The model under review builds one solid part; all positions refer to its coordinate system, in mm. A direction names the side the tool comes from. Coordinates: 2 decimals unless noted, no trailing zeros. Write each loop counter-clockwise with the first axis right and the second up, starting at its lowest first coordinate (ties: lowest second). Pieces come first, ordered by that corner, then holes.
```python
from build123d import *

# Parameters (mm, degrees)
F0_W        = 50
F0_H        = 40
F1_DEPTH    = 8
F2_T        = -1
F3_W        = 15.0767099112
F3_H        = 12.3402951285
F4_DEPTH    = 10
F5_T        = 0.5
F5_T3_DEPTH = 8
F5_T5_DEPTH = 49
F5_T7_DEPTH = 39


# Not quite as in the source:
# - a shell that OpenCascade refuses in one call is made with other operations: the cavity is built on its own and cut out


with BuildPart() as f1:
    # F0 (on Front) → F1 (new body)
    with BuildSketch(Plane.XZ):
        with Locations((-5.8206513731, 0.1503955573)):
            Rectangle(F0_W, F0_H)
    extrude(amount=F1_DEPTH)

    # F2
    f2_openings = [f1.faces().sort_by_distance(p)[0] for p in [
        (-5.820651, 0, 0.150396),
    ]]
    offset(amount=F2_T, openings=f2_openings)

    # F3 (on face) → F4 (join)
    with BuildSketch(Plane(origin=(0, -7, 0), x_dir=(-1, 0, 0), z_dir=(0, 1, 0))):
        with Locations((7.5383549556, -0.1530931331)):
            Rectangle(F3_W, F3_H)
    extrude(amount=F4_DEPTH)

    # F5: shell of thickness 0.5, made by hand


with BuildPart() as f5_core1:
    # F5_t2: copy of F1
    add(f1.part)

    # the walls: a layer under each face that stays
    f5_faces = [f5_core1.faces().sort_by_distance(p)[0] for p in [
        (-5.8206513731, -4, 20.1503955573),
        (19.1793486269, -4, 0.1503955573),
        (-30.8206513731, -4, 0.1503955573),
        (11.3668486269, 0, -19.3557772822),
        (-5.8206513731, -8, 0.1503955573),
        (-5.8206513731, -4, -19.8496044427),
        (-5.8206513731, -3.5, 19.1503955573),
        (18.1793486269, -3.5, 0.1503955573),
        (-5.8206513731, -3.5, -18.8496044427),
        (-29.8206513731, -3.5, 0.1503955573),
        (-21.8206513731, -7, -12.5162711094),
    ]]
    thicken(f5_faces, amount=-F5_T, mode=Mode.SUBTRACT)

    # F5_s4 → F5_t3 (cut)
    with BuildSketch(Plane.XZ.offset(-0.5)):
        Polygon((18.1743486269, 19.1453955573), (18.1793486269, 19.6503955573), (18.6793486269, 19.6503955573), (18.6793486269, 19.1503955573), align=None)
        Polygon((-29.8156513731, 19.1453955573), (-29.8206513731, 19.6503955573), (-30.3206513731, 19.6503955573), (-30.3206513731, 19.1503955573), align=None)
        Polygon((18.1743486269, -18.8446044427), (18.6793486269, -18.8496044427), (18.6793486269, -19.3496044427), (18.1793486269, -19.3496044427), align=None)
        Polygon((-29.8156513731, -18.8446044427), (-29.8206513731, -19.3496044427), (-30.3206513731, -19.3496044427), (-30.3206513731, -18.8496044427), align=None)
    extrude(amount=F5_T3_DEPTH, mode=Mode.SUBTRACT)

    # F5_s6 → F5_t5 (cut)
    with BuildSketch(Plane.YZ.offset(-30.3206513731)):
        Polygon((-6.995, 19.1453955573), (-7, 19.6503955573), (-7.5, 19.6503955573), (-7.5, 19.1503955573), align=None)
        Polygon((-6.995, -18.8446044427), (-7, -19.3496044427), (-7.5, -19.3496044427), (-7.5, -18.8496044427), align=None)
    extrude(amount=F5_T5_DEPTH, mode=Mode.SUBTRACT)

    # F5_s8 → F5_t7 (cut)
    with BuildSketch(Plane.XY.offset(-19.3496044427)):
        Polygon((18.1743486269, -6.995), (18.6793486269, -7), (18.6793486269, -7.5), (18.1793486269, -7.5), align=None)
        Polygon((-29.8156513731, -6.995), (-30.3206513731, -7), (-30.3206513731, -7.5), (-29.8206513731, -7.5), align=None)
    extrude(amount=F5_T7_DEPTH, mode=Mode.SUBTRACT)


with BuildPart() as f1_1:
    add(f1.part)

    # what is left inside the walls is the cavity
    f5_cavity = [f5_core1.part.solids().sort_by_distance(p)[0] for p in [
        (-7.538355, -7.495, -2.209809),
    ]]
    add(f5_cavity, mode=Mode.SUBTRACT)


solid = f1_1.part
```
Item 1: Mouldability with a two-part tool opening along Z and no side actions: class faces 3 (the face through (-6, -3, 19.15)), 4 (the face through (-6, -4, -19.85)), 5 (the face through (-30.821, -4, 0)) as pulls with the +Z half, pulls with the -Z half, needs draft (parallel to the pull), parting line crosses it, or undercut.
Solved:
face 3: undercut
face 4: pulls with the -Z half
face 5: needs draft
Item 2: Take a section at B-B, the plane x = 15.5. Write out the cut boundary in (y, z).
Solved:
outline: (-8, -19.85) - (0, -19.85) - (0, -18.85) - (-7, -18.85) - (-7, 19.15) - (0, 19.15) - (0, 20.15) - (-8, 20.15) - close
Item 3: Take a section at C-C, the plane z = 4. Write out the cut boundary in (x, y), plus the area to 3 significant figures.
Solved:
outline: (-30.82, -8) - (19.18, -8) - (19.18, 0) - (18.18, 0) - (18.18, -7) - (0, -7) - (0, -7.5) - (-15.08, -7.5) - (-15.08, -7) - (-29.82, -7) - (-29.82, 0) - (-30.82, 0) - close
area: 56.5 mm2
Item 4: Machinability: for faces 1 (the face through (-30, 0, 0)), 2 (the face through (-6, -3, -18.85)), which of the approach directions +Z, -Z, +X, -X, +Y, -Y give a long, thin tool a straight path to every point of the face, cutting with its end or side? Answer none if there is none.
Solved:
face 1: +Z, -Z, +X, -X, +Y
face 2: +Y
Item 5: For pin 1 (10 mm diameter, centred on x = -22.5, z = -4, fed in from +Y); pin 2 (6 mm diameter, centred on x = -6, z = 1.5, fed in from +Y), all flat-tipped, find the tip position at first contact; note any pin that passes through.
Solved:
pin 1: stops at y = -7
pin 2: stops at y = -7.5
Item 6: Take a section at A-A, the plane y = -2.5. Write out the cut boundary in (x, z).
Solved:
outline: (-30.82, -19.85) - (19.18, -19.85) - (19.18, 20.15) - (-30.82, 20.15) - close; hole (-29.82, -18.85) - (18.18, -18.85) - (18.18, 19.15) - (-29.82, 19.15) - close
Item 7: To check wall thickness, follow line 1 along Z through (x, y) = (5, -1.25); line 2 along X through (y, z) = (-3.5, -13); line 3 along Y through (x, z) = (1.5, -8.5). State the ranges of each line that lie inside material, in increasing order.
Solved:
line 1: z = -19.85 to -18.85, 19.15 to 20.15
line 2: x = -30.82 to -29.82, 18.18 to 19.18
line 3: y = -8 to -7
Item 8: Take a section at D-D, the plane z = -15. Write out the cut boundary in (x, y).
Solved:
outline: (-30.82, -8) - (19.18, -8) - (19.18, 0) - (18.18, 0) - (18.18, -7) - (-29.82, -7) - (-29.82, 0) - (-30.82, 0) - close
